Here's the drawing with two shaded views (mm, measured from the low corner). I have some questions. Coordinates: 2 decimals unless noted, no trailing zeros. Write each loop counter-clockwise with the first axis right and the second up, starting at its lowest first coordinate (ties: lowest second). Pieces come first, ordered by that corner, then holes. Notation, with made-up numbers: M 26,57 L 68,57 A25 ccw 68,83 Z; hole C 30,-1 d3. An arc over 180 degrees is marked long. Use one line per item in the form item = value. Start each with the question number.
1. I'm going to push flat-ended pins straight in: pin 1 Ø7 at (x, z) = (9, 29.2) entering from +Y; pin 2 Ø9.5 at (y, z) = (62.9, 19.1) entering from +X. Where does each tip first touch, or does it pass through?
2. Please list where these lines run through material, in increasing order: line 1 along X through (y, z) = (111.5, 9); line 2 along Z through (x, y) = (67.2, 13.75); line 3 along X through (y, z) = (19, 10.5). Write a range as [from, to].
3. I want a section at C-C, the plane y = 107. List the corners of the cut face in (x, z) for me.
4. I want a section at A-A, the plane x = 67.2. List the corners of the cut face in (y, z) for me, plus the area to 3 significant figures.
5. I want a section at D-D, the plane z = 29.2. List the corners of the cut face in (x, y) for me, plus the area to 3 significant figures.
6. I want a section at B-B, the plane z = 9. List the corners of the cut face in (x, y) for me, plus the area to 3 significant figures.
7. Thinking about a two-plate mould opening in Z: for the marked faces 1, 2 and 3, which applies, released by +Z, released by -Z, zero draft, split by the parting line, or undercut?
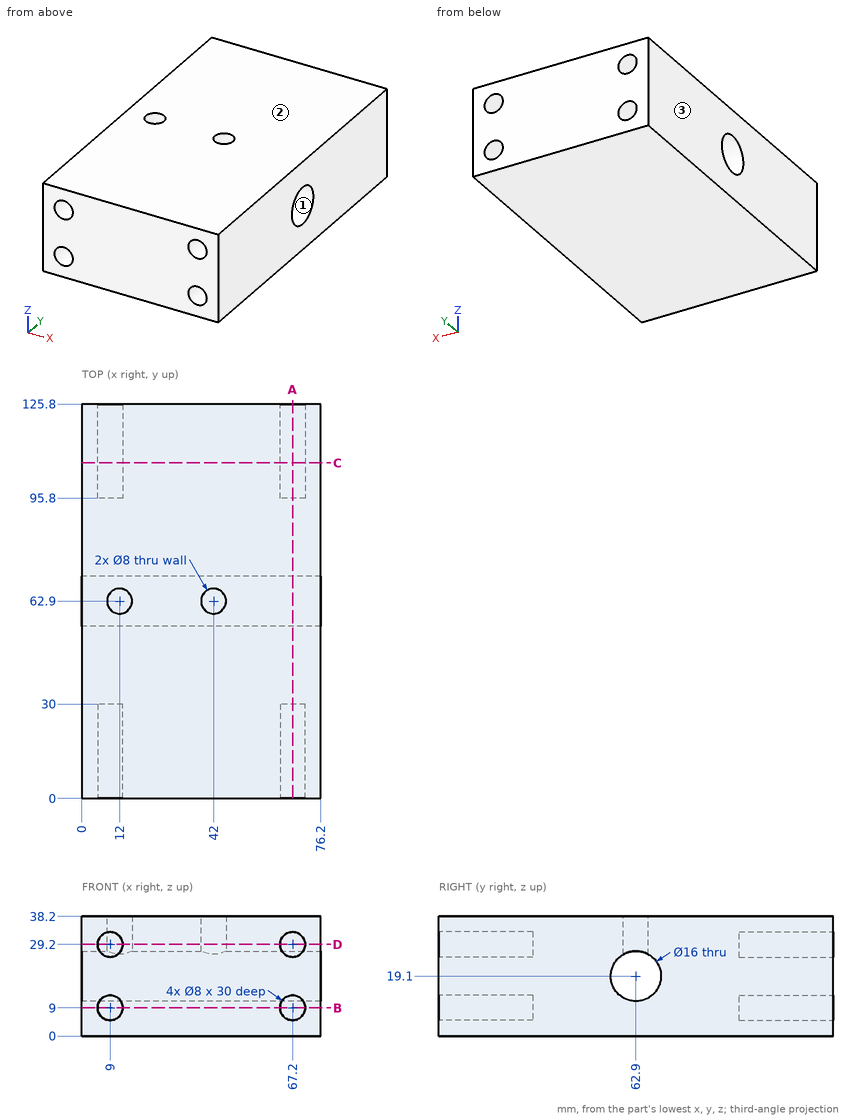
Answer list:
q1.pin_1 = 95.8
q1.pin_2 = through
q2.line_1 = [0, 5], [13, 63.2], [71.2, 76.2]
q2.line_2 = [0, 5], [13, 25.2], [33.2, 38.2]
q2.line_3 = [0, 5.29], [12.71, 63.49], [70.91, 76.2]
q3.outline = M 0,0 L 76.2,0 L 76.2,38.2 L 0,38.2 Z; hole C 9,9 d8; hole C 9,29.2 d8; hole C 67.2,9 d8; hole C 67.2,29.2 d8
q4.outline = M 0,0 L 125.8,0 L 125.8,5 L 95.8,5 L 95.8,13 L 125.8,13 L 125.8,25.2 L 95.8,25.2 L 95.8,33.2 L 125.8,33.2 L 125.8,38.2 L 0,38.2 L 0,33.2 L 30,33.2 L 30,25.2 L 0,25.2 L 0,13 L 30,13 L 30,5 L 0,5 Z; hole C 62.9,19.1 d16
q4.area = 3,640 mm²
q5.outline = M 0,0 L 5,0 L 5,30 L 13,30 L 13,0 L 63.2,0 L 63.2,30 L 71.2,30 L 71.2,0 L 76.2,0 L 76.2,125.8 L 71.2,125.8 L 71.2,95.8 L 63.2,95.8 L 63.2,125.8 L 13,125.8 L 13,95.8 L 5,95.8 L 5,125.8 L 0,125.8 Z; hole C 12,62.9 d8; hole C 42,62.9 d8
q5.area = 8,530 mm²
q6.outline = M 0,0 L 5,0 L 5,30 L 13,30 L 13,0 L 63.2,0 L 63.2,30 L 71.2,30 L 71.2,0 L 76.2,0 L 76.2,125.8 L 71.2,125.8 L 71.2,95.8 L 63.2,95.8 L 63.2,125.8 L 13,125.8 L 13,95.8 L 5,95.8 L 5,125.8 L 0,125.8 Z
q6.area = 8,630 mm²
q7.face_1 = undercut
q7.face_2 = released by +Z
q7.face_3 = zero draft
